Answer from the drawing. Dimensions are ordinates in mm from the lowest x, y and z of the part. Give positions to 0.01 mm unless a question says otherwise; leave off trailing zeros. Loops run counter-clockwise (first coordinate to the right, second up) from the corner with the lowest first, then second, coordinate; pieces in that order, holes last.
(1) Find section A-A, the plane y = 29.5. Write down the section's boundary in (x, z), then the cut area to 3 significant figures.
(2) Find section D-D, the plane y = 20. Write down the section's boundary in (x, z).
(3) This flat-tipped pin is pushed along its axis until it touches: P1, Ø20, axis at x = 42.5, z = 34, coming from the -Y side. Where does it stop, or does it pass through?
(4) Straight lines are drawn through the part: probe 1 along Z at (x, y) = (25, 5); probe 2 along X at (y, z) = (45.5, 21.5); probe 3 along Y at (x, z) = (99.2, 25). For each, find the intervals that lie inside material, in ascending order.
(5) Find section B-B, the plane z = 25. Write down the section's boundary in (x, y).
(6) Determine the mould class of the marked faces 1, 2, 3 and 4 for opening direction Z: pulls with the +Z half, pulls with the -Z half, needs draft (parallel to the pull), parting line crosses it, or undercut.
(7) Find section C-C, the plane x = 64. Write down the section's boundary in (y, z).
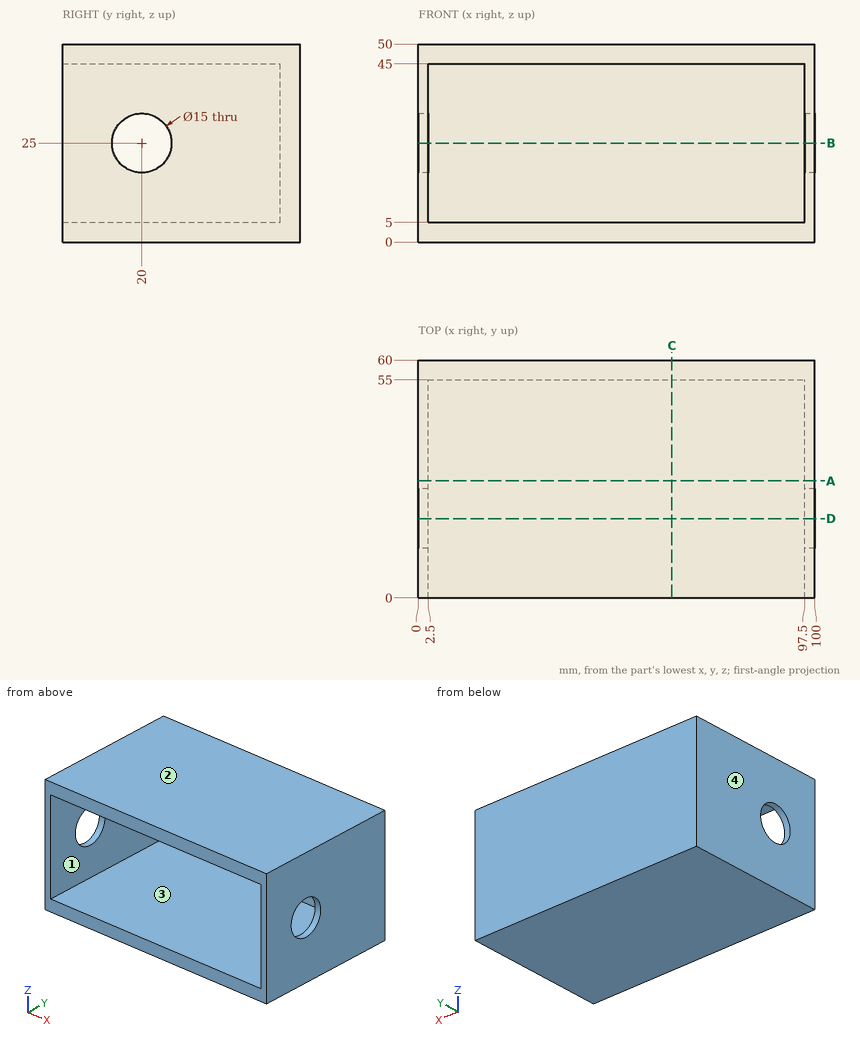
Entries:
1. outline: (0, 0) - (100, 0) - (100, 50) - (0, 50) - close; hole (2.5, 5) - (97.5, 5) - (97.5, 45) - (2.5, 45) - close
1. area: 1,200 mm2
2. outline: (0, 0) - (100, 0) - (100, 17.5) - (97.5, 17.5) - (97.5, 5) - (2.5, 5) - (2.5, 17.5) - (0, 17.5) - close; (0, 32.5) - (2.5, 32.5) - (2.5, 45) - (97.5, 45) - (97.5, 32.5) - (100, 32.5) - (100, 50) - (0, 50) - close
3. P1: stops at y = 55
4. probe 1: z = 0 to 5, 45 to 50
4. probe 2: x = 0 to 2.5, 97.5 to 100
4. probe 3: y = 0 to 12.5, 27.5 to 60
5. outline: (0, 0) - (2.5, 0) - (2.5, 12.5) - (0, 12.5) - close; (0, 27.5) - (2.5, 27.5) - (2.5, 55) - (97.5, 55) - (97.5, 27.5) - (100, 27.5) - (100, 60) - (0, 60) - close; (97.5, 0) - (100, 0) - (100, 12.5) - (97.5, 12.5) - close
6. face 1: undercut
6. face 2: pulls with the +Z half
6. face 3: undercut
6. face 4: needs draft
7. outline: (0, 0) - (60, 0) - (60, 50) - (0, 50) - (0, 45) - (55, 45) - (55, 5) - (0, 5) - close
